Input: part model. Units: mm. Frame: model coordinates. A direction names the side the tool comes from. Give positions to 0.01 mm unless a question says otherwise; leave off trailing zeros. Write each loop counter-clockwise with the first axis right and the second up, starting at its lowest first coordinate (ties: lowest second). Pieces come first, ordered by that corner, then holes. Notation, with made-up numbers: (-3, 79.25) -> (4, 79.25) arc R19 cw to (4, 87.25) -> close; hole circle Ø2 at (-37, 56.25). An arc over 180 degrees is marked (long way). Return JSON: item names as keys, results as strings. Group by question number.
Item 1: Mould query, pull axis X, two halves, no side actions, for faces 1 (the face through (-22.21, 4.96, 53.58)), 2 (the face through (-0.596, 24.587, 2.685)), 3 (the face through (0, 37, 10.607)). Classes: released by +X, released by -X, zero draft, split by the parting line, or undercut.
Item 2: Line query: line 1 (Z direction, x = -34, y = 6); line 2 (X direction, y = 6.4, z = -19); line 3 (X direction, y = 2.1, z = 19). Output: solid intervals per line, ascending. Write a range as [from, to].
Item 3: Pin query (flat end, axial travel): P1, Ø2, axis at x = 39.5, y = 6.5, coming from the -Z side; P2, Ø8, axis at x = 34, z = -17.5, coming from the +Y side; P3, Ø1, axis at y = 4.5, z = -15.5, coming from the -X side; P4, Ø1, axis at x = -7.5, z = -16, coming from the -Y side. Return the tip coordinate at first contact, or that it passes through.
Item 4: Section B-B, the plane y = 20. Return loops of the section in (x, z), then the cut area to 3 significant figures.
Item 5: Set-up query: faces 4 (the face through (0, 2, -4.1)), 5 (the face through (38.88, 7.52, -20.08)), 6 (the face through (-10.607, 37, 0)). Return all of +Z, -Z, +X, -X, +Y, -Y with unobstructed straight access to the full face (end or side cutting, diameter ignored); none if empty.
Item 6: Section C-C, the plane x = -34. Count the separate pieces of the cut face and the enclosed holes in it, then the cut area to 3 significant figures.
from build123d import *

# Parameters (mm, degrees)
SKETCH1_R                      = 58
BOSS_EXTRUDE1_DEPTH            = 10
CBORE_FOR_M5_SHCS3_AT_2_COUNT  = 2
CBORE_FOR_M5_SHCS3_AT_2_PITCH  = 68
CBORE_FOR_M5_SHCS3_AT_3_COUNT  = 2
CBORE_FOR_M5_SHCS3_AT_3_PITCH  = 38
CBORE_FOR_M5_SHCS3_AT_4_COUNT  = 2
CBORE_FOR_M5_SHCS3_AT_4_PITCH  = 77.897368377
SKETCH5_R                      = 20.125
BOSS_EXTRUDE3_DEPTH            = 4
SKETCH4_R                      = 15.1
BOSS_EXTRUDE2_DEPTH            = 15.8
FILLET1_R                      = 2
FILLET2_R                      = 2
SKETCH7_W                      = 21.213203436
SKETCH7_H                      = 21.213203436
BOSS_EXTRUDE4_DEPTH            = 15
M5_CLEARANCE_HOLE1_D           = 5.5
M5_CLEARANCE_HOLE1_CSINK_D     = 5.55
M5_CLEARANCE_HOLE1_CSINK_ANGLE = 90
CUT_EXTRUDE1_DEPTH             = 3.8


with BuildPart() as part:
    # Sketch1 → Boss-Extrude1 (new body)
    with BuildSketch(Plane(origin=(0, 0, 0), x_dir=(1, 0, 0), z_dir=(0, 1, 0))):
        with Locations(Location((0, 0, 0), (0, 0, 270))):
            Circle(SKETCH1_R)
    extrude(amount=BOSS_EXTRUDE1_DEPTH)

    # Sketch3 → CBORE for M5 SHCS3 (revolve, cut)
    with BuildSketch(Plane(origin=(-34, 10, -19), x_dir=(0, 0, 1), z_dir=(1, 0, 0))):
        Polygon((0, 0), (0, 10), (2.75, 10), (2.75, 5), (5, 5), (5, 0.025), (5.025, 0), align=None)
    cbore_for_m5_shcs3 = revolve(axis=Axis((-34, 16.35, -19), (0, -1, 0)), mode=Mode.SUBTRACT)

    # CBORE for M5 SHCS3 at 2: CBORE for M5 SHCS3 ×2
    with Locations(*[(i * CBORE_FOR_M5_SHCS3_AT_2_PITCH, 0, 0) for i in range(1, CBORE_FOR_M5_SHCS3_AT_2_COUNT)]):
        add(cbore_for_m5_shcs3, mode=Mode.SUBTRACT)

    # CBORE for M5 SHCS3 at 3: CBORE for M5 SHCS3 ×2
    with Locations(*[(0, 0, i * CBORE_FOR_M5_SHCS3_AT_3_PITCH) for i in range(1, CBORE_FOR_M5_SHCS3_AT_3_COUNT)]):
        add(cbore_for_m5_shcs3, mode=Mode.SUBTRACT)

    # CBORE for M5 SHCS3 at 4: CBORE for M5 SHCS3 ×2
    with Locations(*[Vector(0.8729434821372646, 0, 0.48782135766494195) * (i * CBORE_FOR_M5_SHCS3_AT_4_PITCH) for i in range(1, CBORE_FOR_M5_SHCS3_AT_4_COUNT)]):
        add(cbore_for_m5_shcs3, mode=Mode.SUBTRACT)

    # Sketch5 → Boss-Extrude3 (add)
    with BuildSketch(Plane(origin=(0, 10, 0), x_dir=(1, 0, 0), z_dir=(0, 1, 0))):
        with Locations(Location((0, 0, 0), (0, 0, 270))):
            Circle(SKETCH5_R)
    extrude(amount=BOSS_EXTRUDE3_DEPTH)

    # Sketch4 → Boss-Extrude2 (add)
    with BuildSketch(Plane(origin=(0, 14, 0), x_dir=(1, 0, 0), z_dir=(0, 1, 0))):
        with Locations(Location((0, 0, 0), (0, 0, 270))):
            Circle(SKETCH4_R)
    extrude(amount=BOSS_EXTRUDE2_DEPTH)

    # Fillet1
    fillet1_edges = [part.edges().sort_by_distance(p)[0] for p in [
        (0, 0, -58),
        (0, 10, -58),
    ]]
    fillet(fillet1_edges, radius=FILLET1_R)

    # Fillet2
    fillet2_edges = [part.edges().sort_by_distance(p)[0] for p in [
        (0, 10, -20.125),
    ]]
    fillet(fillet2_edges, radius=FILLET2_R)

    # Sketch7 → Boss-Extrude4 (add)
    with BuildSketch(Plane(origin=(0, 29.8, 0), x_dir=(1, 0, 0), z_dir=(0, 1, 0))):
        Rectangle(SKETCH7_W, SKETCH7_H)
    extrude(amount=BOSS_EXTRUDE4_DEPTH)

    # M5 Clearance Hole1 (through all)
    with Locations(Plane(origin=(0, 0, 0), x_dir=(-1, 0, 0), z_dir=(0, -1, 0))):
        with Locations((0, 0)):
            CounterSinkHole(M5_CLEARANCE_HOLE1_D / 2, M5_CLEARANCE_HOLE1_CSINK_D / 2, counter_sink_angle=M5_CLEARANCE_HOLE1_CSINK_ANGLE)

    # Sketch10 → Cut-Extrude1 (cut)
    with BuildSketch(Plane.XZ):
        Polygon((2.367136104, 4.1), (-2.367136104, 4.1), (-4.734272207, 0), (-2.367136104, -4.1), (2.367136104, -4.1), (4.734272207, 0), align=None)
    extrude(amount=-CUT_EXTRUDE1_DEPTH, mode=Mode.SUBTRACT)


solid = part.part
Answer below:
{
 "1": {"face 1": "split by the parting line", "face 2": "undercut", "face 3": "zero draft"},
 "2": {"line 1": "z = [-46.99, -24], [-14, 14], [24, 46.99]", "line 2": "x = [-54.8, -39], [-29, 29], [39, 54.8]", "line 3": "x = [-54.8, -36.75], [-31.25, 31.25], [36.75, 54.8]"},
 "3": {"P1": "stops at z = -43.38", "P2": "stops at y = 10", "P3": "stops at x = -56.03", "P4": "stops at y = 0"},
 "4": {"outline": "circle Ø30.2 at (0, 0); hole circle Ø5.5 at (0, 0)", "area": "693 mm2"},
 "5": {"face 4": "-Y", "face 5": "+Y", "face 6": "+Z, -Z, -X, +Y"},
 "6": {"separate pieces": "3", "enclosed holes": "0", "area": "781 mm2"}
}
